Here's how the part is built. I have some questions about the finished solid (model axes, mm). A direction names the side the tool comes from. Round coordinates to 2 decimals unless told otherwise and drop trailing zeros. Write each loop counter-clockwise with the first axis right and the second up, starting at its lowest first coordinate (ties: lowest second). Pieces come first, ordered by that corner, then holes. Notation, with made-up numbers: (36.5, 16.25) - (73.5, 16.25) arc R34 ccw to (73.5, 53.25) - close; hole circle Ø11 at (-7.75, 7.25). An arc over 180 degrees is marked (long way). One line per question, with ' | ' between items. Start each with the question number.
(1) For faces 1 (the flat face through (3.3, 0, -0.1)), 2 (the flat face through (0.76, -3, 0)), which set-ups out of +Z, -Z, +X, -X, +Y, -Y let a thin tool reach every point of the face, with its end or its side?
(2) Thinking about a two-plate mould opening in X: for faces 3 (the flat face through (-0.76, -3, 0)), 4 (the flat face through (0, 20, 0)), 5 (the cylindrical face through (0.9, 9.61, 2.86)), 6 (the flat face through (0, -2.29, 0)), which applies, pulls with the +X half, pulls with the -X half, needs draft (parallel to the pull), parting line crosses it, or undercut?
(3) Will these pins go through, and if not, where does the flat tip stop? pin 1 (1 mm diameter, centred on x = 2.5, z = -0.5, fed in from +Y); pin 2 (3 mm diameter, centred on y = 10.5, z = 3.5, fed in from +X); pin 3 (1.5 mm diameter, centred on y = 12, z = -3.5, fed in from +X); pin 4 (2 mm diameter, centred on y = -3.5, z = -0.5, fed in from +X).
(4) If I drill on L1, parallel to X at y = 4.25, z = -0.5; L2, parallel to Y at x = -1.75, z = -4; L3, parallel to X at y = -0.25, z = 2.5, over which ranges is the centre line in solid material (lowest first)?
(5) Imagine slicing it at A-A (y = 8.5). Write out the boundary of the cut face in (x, z).
from build123d import *

# Parameters (mm, degrees)
SKETCH1_R               = 3
BOSS_EXTRUDE1_DEPTH     = 20
CHAMFER1_SIZE           = 0.5
CUT_EXTRUDE1_DEPTH      = 22.213203483
CUT_EXTRUDE1_DEPTH_BACK = 22.213203483


with BuildPart() as part:
    # Sketch1 → Boss-Extrude1 (new body)
    with BuildSketch(Plane(origin=(0, 0, 0), x_dir=(1, 0, 0), z_dir=(0, 1, 0))):
        with Locations(Location((0, 0, 0), (0, 0, 270))):
            Circle(SKETCH1_R)
    extrude(amount=BOSS_EXTRUDE1_DEPTH)

    # Chamfer1
    chamfer1_edges = [part.edges().sort_by_distance(p)[0] for p in [
        (0, 20, -3),
    ]]
    chamfer(chamfer1_edges, length=CHAMFER1_SIZE)

    # Sketch2 → Revolve1 (revolve)
    with BuildSketch(Plane.XY, mode=Mode.PRIVATE) as revolve1_sk:
        with BuildLine():
            Line((0, 0), (-5, 0))
            ThreePointArc((-5, 0), (-3.260312474, -3.005133898), (0, -4.2))
            Line((0, -4.2), (0, 0))
        make_face()
    revolve(revolve1_sk.sketch.rotate(Axis((0, -4.2, 0), (0, 1, 0)), 270), axis=Axis((0, -4.2, 0), (0, 1, 0)))

    # Sketch3 → Cut-Extrude1 (cut, two sides: drawn at the far end of the back side and taken through both)
    with BuildSketch(Plane.XY.offset(-CUT_EXTRUDE1_DEPTH_BACK)):
        Polygon((-0.76031497, -2.29), (0, -2.29), (0.76031497, -2.29), (0.76031497, -6.2280618), (-0.76031497, -6.2280618), align=None)
    extrude(amount=CUT_EXTRUDE1_DEPTH + CUT_EXTRUDE1_DEPTH_BACK, mode=Mode.SUBTRACT)


solid = part.part
Check sheet entries:
1) face 1: +Y | face 2: +Z, -Z, -Y
2) face 3: undercut | face 4: needs draft | face 5: parting line crosses it | face 6: undercut
3) pin 1: y = 20 | pin 2: x = 2.24 | pin 3: x = 1.2 | pin 4: x = 3.76
4) L1: -2.96 to 2.96 | L2: -1.7 to 0 | L3: -4.27 to 4.27
5) outline: circle Ø6 at (0, 0)
